from build123d import *

# Parameters (mm, degrees)
F0_W      = 9.4
F0_H      = 3.61
F1_DEPTH  = 10.47
F2_R      = 1
F3_W      = 4.6
F3_H      = 1
F3_H_2    = 0.805
F4_DEPTH  = 0.25
F6_DEPTH  = 0.25
F8_DEPTH  = 5
F9_W      = 0.1
F9_H      = 0.1
F10_DEPTH = 3.6


with BuildPart() as f1:
    # F0 (on Front) → F1 (new body)
    with BuildSketch(Plane.XZ):
        with Locations((-0.355073555, 5.140078254)):
            Rectangle(F0_W, F0_H)
    extrude(amount=F1_DEPTH)

    # F2
    f2_edges = [f1.edges().sort_by_distance(p)[0] for p in [
        (4.344926, -5.235, 6.945078),
        (4.344926, -5.235, 3.335078),
        (-5.055074, -5.235, 6.945078),
        (-5.055074, -5.235, 3.335078),
    ]]
    fillet(f2_edges, radius=F2_R)

    # F3 (on face) → F4 (join)
    with BuildSketch(Plane.YZ.offset(4.344926445)):
        Polygon((-2.72, -0.264921746), (-2.72, 3.335078254), (-7.32, 3.335078254), (-7.32, 1.135078254), (-6.82, 1.135078254), (-6.82, -0.264921746), (-5.62, -0.264921746), (-5.62, 1.135078254), (-5.12, 1.135078254), (-5.12, 1.635078254), (-3.62, 1.635078254), (-3.62, -0.264921746), align=None)
        with Locations((-5.02, 3.835078254)):
            Rectangle(F3_W, F3_H)
        with Locations((-5.02, 4.737578254)):
            Rectangle(F3_W, F3_H_2)
    extrude(amount=-F4_DEPTH)

    # F5 (on face) → F6 (join)
    with BuildSketch(Plane(origin=(-5.055073555, 0, 0), x_dir=(0, -1, 0), z_dir=(-1, 0, 0))):
        Polygon((7.32, 1.135078254), (7.32, 4.335078254), (2.72, 4.335078254), (2.72, -0.264921746), (3.62, -0.264921746), (3.62, 1.635078254), (5.12, 1.635078254), (5.12, 1.135078254), (5.62, 1.135078254), (5.62, -0.264921746), (6.82, -0.264921746), (6.82, 1.135078254), align=None)
    extrude(amount=-F6_DEPTH)

    # F7 (on face) → F8 (cut)
    with BuildSketch(Plane.XZ.offset(10.47)):
        with BuildLine():
            Line((3.344926445, 6.645078254), (-4.055073555, 6.645078254))
            ThreePointArc((-4.055073555, 6.645078254), (-4.5500483018, 6.4400530009), (-4.755073555, 5.945078254))
            Line((-4.755073555, 5.945078254), (-4.755073555, 4.335078254))
            ThreePointArc((-4.755073555, 4.335078254), (-4.5500483018, 3.8401035072), (-4.055073555, 3.635078254))
            Line((-4.055073555, 3.635078254), (3.344926445, 3.635078254))
            ThreePointArc((3.344926445, 3.635078254), (3.8399011918, 3.8401035072), (4.044926445, 4.335078254))
            Line((4.044926445, 4.335078254), (4.044926445, 5.945078254))
            ThreePointArc((4.044926445, 5.945078254), (3.8399011918, 6.4400530009), (3.344926445, 6.645078254))
        make_face()
    extrude(amount=-F8_DEPTH, mode=Mode.SUBTRACT)

    # F9 (on face) → F10 (join, through all)
    with BuildSketch(Plane(origin=(0, 0, 3.335078254), x_dir=(1, 0, 0), z_dir=(0, 0, -1))):
        with Locations((-3.155073555, 1.9)):
            Rectangle(F9_W, F9_H)
        with Locations((-1.555073555, 1.9)):
            Rectangle(F9_W, F9_H)
        Polygon((-0.705073555, 1.95), (-0.805073555, 1.95), (-0.805073555, 1.85), (-0.705073555, 1.85), (-0.705073555, 1.9), align=None)
        Polygon((-0.005073555, 1.95), (-0.005073555, 1.9), (-0.005073555, 1.85), (0.094926445, 1.85), (0.094926445, 1.95), align=None)
        Polygon((-1.105073555, 2.85), (-1.205073555, 2.85), (-1.205073555, 2.75), (-1.105073555, 2.75), (-1.105073555, 2.8), align=None)
        with Locations((-1.955073555, 2.8)):
            Rectangle(F9_W, F9_H)
        with Locations((-2.755073555, 2.8)):
            Rectangle(F9_W, F9_H)
        Polygon((0.394926445, 2.85), (0.394926445, 2.8), (0.394926445, 2.75), (0.494926445, 2.75), (0.494926445, 2.85), align=None)
        with Locations((0.844926445, 1.9)):
            Rectangle(F9_W, F9_H)
        with Locations((1.244926445, 2.8)):
            Rectangle(F9_W, F9_H)
        with Locations((2.044926445, 2.8)):
            Rectangle(F9_W, F9_H)
        with Locations((2.444926445, 1.9)):
            Rectangle(F9_W, F9_H)
    extrude(amount=F10_DEPTH)


solid = f1.part
CAD build for the part. Positions are in the model's coordinates, mm. A direction names the side the tool comes from. Round coordinates to 2 decimals unless told otherwise and drop trailing zeros. Loops run counter-clockwise (first coordinate to the right, second up) from the corner with the lowest first, then second, coordinate; pieces in that order, holes last. Notation, with made-up numbers: (-32.75, 45) - (15.25, 45) arc R5 ccw to (15.25, 54) - close; hole circle Ø6 at (-5, 75). An arc over 180 degrees is marked (long way). Put each result on its own line as item: value.
1. Slice it at C-C on x = -3.5. List the corners of the cut face in (y, z).
Geometry check:
outline: (-10.47, 3.34) - (0, 3.34) - (0, 6.95) - (-10.47, 6.95) - (-10.47, 6.65) - (-5.47, 6.65) - (-5.47, 3.64) - (-10.47, 3.64) - close
2. 3-axis set-ups, long thin cutter, end or side, ignore diameter. For faces 4 (the cylindrical face through (4.1, -5.3, 6.6)), 5 (the flat face through (0, -5.47, 5)), 6 (the flat face through (-4.805, -5, 2)): which of +Z, -Z, +X, -X, +Y, -Y reach the whole face in a straight line?
Geometry check:
face 4: +Z, +X, +Y, -Y
face 5: -Y
face 6: -Z, +Y, -Y
3. Pin check, flat tip, straight feed: P1, Ø1, axis at y = -8, z = 2.5, coming from the +X side. Stop position of the tip, or through.
Geometry check:
P1: through
4. Wall check: line 1 (Z direction, x = -1.25, y = -5.75); line 2 (X direction, y = -6.25, z = 4.5); line 3 (Z direction, x = -2, y = -4). Give the ranges that are in metal, low to high.
Geometry check:
line 1: 3.34 to 3.64, 6.65 to 6.95
line 2: -5.06 to -4.76, 4.04 to 4.34
line 3: 3.34 to 6.95
5. Slice it at A-A on y = -5.75. List the corners of the cut face in (x, z).
Geometry check:
outline: (-5.06, -0.26) - (-4.81, -0.26) - (-4.81, 3.67) arc R1 ccw to (-4.06, 3.34) - (3.34, 3.34) arc R1 ccw to (4.09, 3.67) - (4.09, -0.26) - (4.34, -0.26) - (4.34, 5.95) arc R1 ccw to (3.34, 6.95) - (-4.06, 6.95) arc R1 ccw to (-5.06, 5.95) - close; hole (-4.76, 4.34) arc R0.7 ccw to (-4.06, 3.64) - (3.34, 3.64) arc R0.7 ccw to (4.04, 4.34) - (4.04, 5.95) arc R0.7 ccw to (3.34, 6.65) - (-4.06, 6.65) arc R0.7 ccw to (-4.76, 5.95) - close
6. Two-plate mould, pull along Z, no slides. Class faces 1 (the flat face through (4.045, -8, 5)), 2 (the flat face through (4.095, -5, 2)), 3 (the flat face through (0, -5, 6.945)): released by +Z, released by -Z, zero draft, split by the parting line, or undercut.
Geometry check:
face 1: undercut
face 2: zero draft
face 3: released by +Z
7. Slice it at B-B on y = -4.5. List the corners of the cut face in (x, z), and give its area (3 significant figures).
Geometry check:
outline: (-5.06, 1.64) - (-4.81, 1.64) - (-4.81, 3.67) arc R1 ccw to (-4.06, 3.34) - (3.34, 3.34) arc R1 ccw to (4.09, 3.67) - (4.09, 1.64) - (4.34, 1.64) - (4.34, 5.95) arc R1 ccw to (3.34, 6.95) - (-4.06, 6.95) arc R1 ccw to (-5.06, 5.95) - close
area: 34.2 mm²
8. Slice it at D-D on z = 6.25. List the corners of the cut face in (x, y), and give its area (3 significant figures).
Geometry check:
outline: (-5.01, -10.47) - (-4.69, -10.47) - (-4.69, -5.47) - (3.98, -5.47) - (3.98, -10.47) - (4.3, -10.47) - (4.3, 0) - (-5.01, 0) - close
area: 54.1 mm²
